Autodesk Inventor part; units mm, degrees
ref_plane "YZ Plane" through (0, 0, 0) normal (1, 0, 0) x (0, 1, 0)
ref_plane "XZ Plane" through (0, 0, 0) normal (0, 1, 0) x (-1, 0, 0)
ref_plane "XY Plane" through (0, 0, 0) normal (0, 0, 1) x (1, 0, 0)
sketch "Sketch1" plane through (0, 0, 0) normal (0, 0, 1) x (1, 0, 0)
  circle A0 centre (0, 0) radius 195 construction
  circle A1 centre (0, 0) radius 205
  circle A2 centre (0, 0) radius 63
  dimension "d0" = 390
  dimension "d4" = 126
  dimension "d13" = 10
extrude "Extrusion1" add sketch "Sketch1" along normal blind 10
sketch "Sketch3" plane through (0, 0, 0) normal (0, 0, -1) x (-1, 0, 0)
  circle A0 centre (0, 0) radius 205 construction
  circle A1 centre (-187.6666, -82.5) radius 2.5
  circle A2 centre (187.6666, -82.5) radius 2.5
  line L0 (-187.6666, -82.5) -> (187.6666, -82.5) construction
  dimension "d14" = 5
  dimension "d15" = 82.5
extrude "Extrusion3" cut sketch "Sketch3" against normal through all
equation "\"d0\" = Шпил_пласт_НОС_диам_центров"
equation "\"d4\" = Стенка_НОС_диам_илоотвод"
equation "\"d2\" = Thickness"
equation "\"BendReliefDepth\" = 0.5 * Thickness"
properties part number "ДМФ 032 крышка Нос"
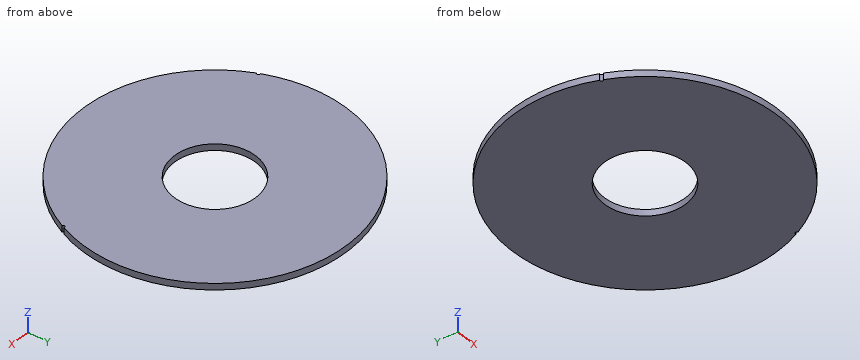
For this review, take the finished solid that the model builds, in its own axes (mm). Round coordinates to 2 decimals unless told otherwise and drop trailing zeros. Write each loop counter-clockwise with the first axis right and the second up, starting at its lowest first coordinate (ties: lowest second). Pieces come first, ordered by that corner, then holes.
1) Take a section at C-C on z = 3. Give the boundary of the cut face in (x, y).
Answer below:
outline: (-188.66, -80.21) arc R2.5 cw to (-186.65, -84.78) arc R205 ccw to (186.65, -84.78) arc R2.5 cw to (188.66, -80.21) arc R205 ccw (long way) to start; hole circle Ø126 at (0, 0)
2) Take a section at D-D on y = 150. Give the boundary of the cut face in (x, z), then the cut area to 3 significant figures.
Answer below:
outline: (-139.73, 0) - (139.73, 0) - (139.73, 10) - (-139.73, 10) - close
area: 2,790 mm2
3) For line 1 along Y through (x, z) = (0, 4.5); line 2 along X through (y, z) = (-56, 8.25); line 3 along Y through (x, z) = (-41, 8), list the stretches that pass through material, from the lowest coordinate up.
Answer below:
line 1: y = -205 to -63, 63 to 205
line 2: x = -197.2 to -28.86, 28.86 to 197.2
line 3: y = -200.86 to -47.83, 47.83 to 200.86
4) Insertion check: pin 1 Ø6 at (y, z) = (27.5, 4.5) entering from -X; pin 2 Ø4 at (x, z) = (129, 5) entering from -Y; pin 3 Ø3 at (x, z) = (51.5, 9) entering from -Y. Each pin has a flat end and moves straight along its axis. Give the tip position at first contact, or say it passes through.
Answer below:
pin 1: stops at x = -203.53
pin 2: stops at y = -160.92
pin 3: stops at y = -198.81
5) Take a section at B-B on y = 40. Give the boundary of the cut face in (x, z), then the cut area to 3 significant figures.
Answer below:
outline: (-201.06, 0) - (-48.67, 0) - (-48.67, 10) - (-201.06, 10) - close; (48.67, 0) - (201.06, 0) - (201.06, 10) - (48.67, 10) - close
area: 3,050 mm2
6) Take a section at A-A on x = 0. Give the boundary of the cut face in (y, z).
Answer below:
outline: (-205, 0) - (-63, 0) - (-63, 10) - (-205, 10) - close; (63, 0) - (205, 0) - (205, 10) - (63, 10) - close
